CAD build for the part. Positions are in the model's coordinates, mm. A direction names the side the tool comes from. Coordinates: 2 decimals unless noted, no trailing zeros. Order: outer loops, then holes, each group sorted by start corner. A loop starts at its lowest first (then second) coordinate and runs counter-clockwise, first axis right, second up.
from build123d import *

# Parameters (mm, degrees)
BOSS_EXTRUDE1_DEPTH = 16.51
SKETCH2_R           = 11.3665
SKETCH2_R_2         = 3.175
BOSS_EXTRUDE2_DEPTH = 6.223
SKETCH3_W           = 1.27
SKETCH3_H           = 3.175
SKETCH4_R           = 3.175
CUT_EXTRUDE1_DEPTH  = 54.61


with BuildPart() as part:
    # Sketch1 → Boss-Extrude1 (new body, symmetric)
    with BuildSketch(Plane.XY):
        with BuildLine():
            Line((-28.829, 11.938), (-27.559, 11.938))
            ThreePointArc((-27.559, 11.938), (-26.62906403, 9.69293597), (-24.384, 8.763))
            Line((-24.384, 8.763), (-11.176, 8.763))
            Line((-11.176, 8.763), (-11.176, 55.245))
            Line((-11.176, 55.245), (0, 55.245))
            Line((0, 55.245), (0, 0))
            Line((0, 0), (-25.019, 0))
            ThreePointArc((-25.019, 0), (-27.713076836, 1.115923164), (-28.829, 3.81))
            Line((-28.829, 3.81), (-28.829, 11.938))
        make_face()
    extrude(amount=BOSS_EXTRUDE1_DEPTH, both=True)

    # Sketch2 → Boss-Extrude2 (add)
    with BuildSketch(Plane(origin=(0, 0, 0), x_dir=(0, 0, -1), z_dir=(1, 0, 0))):
        with Locations((0, 42.418)):
            Circle(SKETCH2_R)
        with Locations((0, 42.418)):
            Circle(SKETCH2_R_2, mode=Mode.SUBTRACT)
        with BuildLine():
            Line((-0.8255, 48.521932339), (-0.8255, 51.715926651))
            ThreePointArc((-0.8255, 51.715926651), (-4.66725, 50.501914132), (-7.639490682, 47.781867296))
            Line((-7.639490682, 47.781867296), (-4.873410469, 46.18487014))
            ThreePointArc((-4.873410469, 46.18487014), (-3.07975, 47.752283475), (-0.8255, 48.521932339))
        make_face(mode=Mode.SUBTRACT)
        with BuildLine():
            Line((0.8255, 48.521932339), (0.8255, 51.715926651))
            ThreePointArc((0.8255, 51.715926651), (4.66725, 50.501914132), (7.639490682, 47.781867296))
            Line((7.639490682, 47.781867296), (4.873410469, 46.18487014))
            ThreePointArc((4.873410469, 46.18487014), (3.07975, 47.752283475), (0.8255, 48.521932339))
        make_face(mode=Mode.SUBTRACT)
        with BuildLine():
            Line((5.698910469, 44.755062199), (8.464990682, 46.352059354))
            ThreePointArc((8.464990682, 46.352059354), (9.3345, 42.418), (8.464990682, 38.483940646))
            Line((8.464990682, 38.483940646), (5.698910469, 40.080937801))
            ThreePointArc((5.698910469, 40.080937801), (6.1595, 42.418), (5.698910469, 44.755062199))
        make_face(mode=Mode.SUBTRACT)
        with BuildLine():
            Line((4.873410469, 38.65112986), (7.639490682, 37.054132704))
            ThreePointArc((7.639490682, 37.054132704), (4.66725, 34.334085868), (0.8255, 33.120073349))
            Line((0.8255, 33.120073349), (0.8255, 36.314067661))
            ThreePointArc((0.8255, 36.314067661), (3.07975, 37.083716525), (4.873410469, 38.65112986))
        make_face(mode=Mode.SUBTRACT)
        with BuildLine():
            Line((-0.8255, 36.314067661), (-0.8255, 33.120073349))
            ThreePointArc((-0.8255, 33.120073349), (-4.66725, 34.334085868), (-7.639490682, 37.054132704))
            Line((-7.639490682, 37.054132704), (-4.873410469, 38.65112986))
            ThreePointArc((-4.873410469, 38.65112986), (-3.07975, 37.083716525), (-0.8255, 36.314067661))
        make_face(mode=Mode.SUBTRACT)
        with BuildLine():
            Line((-5.698910469, 40.080937801), (-8.464990682, 38.483940646))
            ThreePointArc((-8.464990682, 38.483940646), (-9.3345, 42.418), (-8.464990682, 46.352059354))
            Line((-8.464990682, 46.352059354), (-5.698910469, 44.755062199))
            ThreePointArc((-5.698910469, 44.755062199), (-6.1595, 42.418), (-5.698910469, 40.080937801))
        make_face(mode=Mode.SUBTRACT)
    extrude(amount=BOSS_EXTRUDE2_DEPTH)

    # Sketch3 → Cut-Revolve1 (revolve, cut)
    with BuildSketch(Plane.XY):
        with Locations((5.588, 50.165)):
            Rectangle(SKETCH3_W, SKETCH3_H)
    revolve(axis=Axis((6.223, 42.418, 0), (-1, 0, 0)), mode=Mode.SUBTRACT)

    # Sketch4 → Cut-Extrude1 (cut)
    with BuildSketch(Plane(origin=(0, 55.245, 0), x_dir=(1, 0, 0), z_dir=(0, 1, 0))):
        with BuildLine():
            Line((-1.651, 3.965573729), (-1.651, 14.859))
            Line((-1.651, 14.859), (-9.525, 14.859))
            Line((-9.525, 14.859), (-9.525, 3.965573729))
            ThreePointArc((-9.525, 3.965573729), (-5.588, 5.588), (-1.651, 3.965573729))
        make_face()
        with BuildLine():
            Line((-1.651, -14.859), (-1.651, -3.965573729))
            ThreePointArc((-1.651, -3.965573729), (-5.588, -5.588), (-9.525, -3.965573729))
            Line((-9.525, -3.965573729), (-9.525, -14.859))
            Line((-9.525, -14.859), (-1.651, -14.859))
        make_face()
        with Locations((-5.588, 0)):
            Circle(SKETCH4_R)
    extrude(amount=-CUT_EXTRUDE1_DEPTH, mode=Mode.SUBTRACT)


solid = part.part
1) Slice it at D-D (z = 13.5). List the corners of the cut face in (x, y) (3 decimals), plus the area to 3 significant figures.
2) Which spindle directions (+Z, -Z, +X, -X, +Y, -Y) get a long thin tool onto all of the face, cutting with end or side? Do faces 4 (the flat face through (-18, 8.763, 0)), 5 (the flat face through (-28, 11.938, 0)), 6 (the flat face through (2.442, 39.294, 7.063)). Say none if no direction does.
3) Slice it at A-A (y = 10). List the corners of the cut face in (x, z) (3 decimals).
4) Slice it at C-C (x = -6.5). List the corners of the cut face in (y, z) (3 decimals).
5) Pin check, flat tips, straight feed: P1, Ø10.5, axis at x = -19, z = -0.5, coming from the +Y side; P2, Ø10, axis at x = -21.5, z = -11, coming from the -Y side; P3, Ø1.3, axis at y = 50.5, z = 0, coming from the +X side; P4, Ø1, axis at x = -28.5, z = 6.5, coming from the +Y side. Stop position of each tip, or through.
6) Drill centre lines: probe 1 along X at (y, z) = (28.5, -11) (3 decimals); probe 2 along Z at (x, y) = (-6, 43); probe 3 along X at (y, z) = (11, 7.5) (3 decimals). Where is each one in solid material? Low to high.
7) Two-plate mould, pull along X, no slides. Class faces 1 (the flat face through (2, 38, 6)), 2 (the cylindrical face through (-5.527, 28.322, 5.588)), 3 (the flat face through (0, 36, -4)): released by +X, released by -X, zero draft, split by the parting line, or undercut.
Worked out:
1. outline: (-28.829, 3.81) arc R3.81 ccw to (-25.019, 0) - (0, 0) - (0, 55.245) - (-1.651, 55.245) - (-1.651, 0.635) - (-9.525, 0.635) - (-9.525, 55.245) - (-11.176, 55.245) - (-11.176, 8.763) - (-24.384, 8.763) arc R3.175 cw to (-27.559, 11.938) - (-28.829, 11.938) - close
1. area: 345 mm2
2. face 4: +Z, -Z, +Y
2. face 5: +Z, -Z, -X, +Y
2. face 6: +X
3. outline: (-28.829, -16.51) - (-26.899, -16.51) - (-26.899, 16.51) - (-28.829, 16.51) - close; (-11.176, -16.51) - (0, -16.51) - (0, 16.51) - (-11.176, 16.51) - close; hole (-9.525, -14.859) - (-1.651, -14.859) - (-1.651, -3.966) arc R5.588 cw to (-9.525, -3.966) - close; hole (-9.525, 3.966) arc R5.588 cw to (-1.651, 3.966) - (-1.651, 14.859) - (-9.525, 14.859) - close; hole circle Ø6.35 at (-5.588, 0)
4. outline: (0, -16.51) - (55.245, -16.51) - (55.245, -14.859) - (0.635, -14.859) - (0.635, -5.513) - (55.245, -5.513) - (55.245, -3.041) - (0.635, -3.041) - (0.635, 3.041) - (55.245, 3.041) - (55.245, 5.513) - (0.635, 5.513) - (0.635, 14.859) - (55.245, 14.859) - (55.245, 16.51) - (0, 16.51) - close
5. P1: stops at y = 8.76
5. P2: stops at y = 0
5. P3: stops at x = 4.95
5. P4: stops at y = 11.94
6. probe 1: x = -11.176 to -9.525, -1.651 to 0
6. probe 2: z = -16.51 to -14.86, -5.57 to -3.15, 3.15 to 5.57, 14.86 to 16.51
6. probe 3: x = -28.829 to -27.417, -11.176 to -9.525, -1.651 to 0
7. face 1: zero draft
7. face 2: undercut
7. face 3: released by +X
